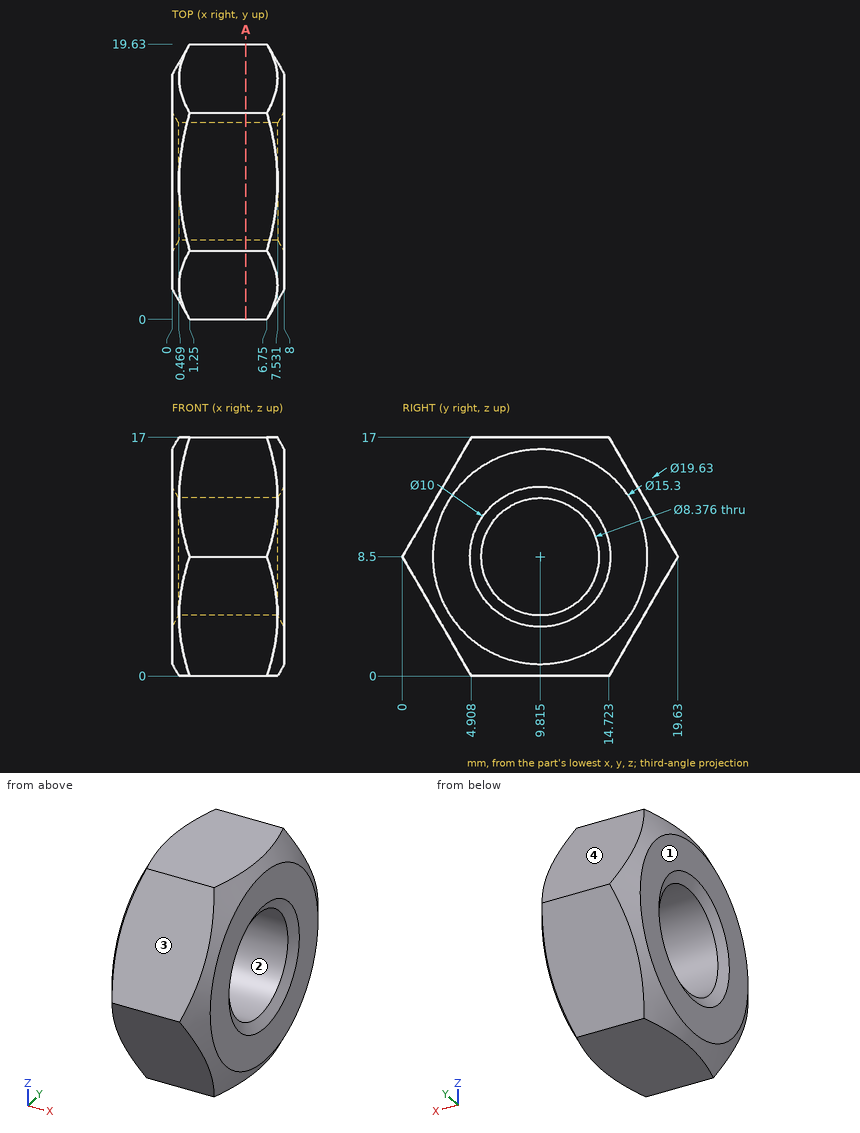
Geometry: see drawing. Coordinates: mm, zero at the bounding-box minimum. Coordinates: 2 decimals unless noted, no trailing zeros. Loops run counter-clockwise (first coordinate to the right, second up) from the corner with the lowest first, then second, coordinate; pieces in that order, holes last. Notation, with made-up numbers: (60.5, -4.5) - (88.5, -4.5) arc R28 cw to (88.5, 29.5) - close; hole circle Ø4 at (44, 46.5). An arc over 180 degrees is marked (long way). Answer in a Markdown table with one row per item.
(1) Pin query (flat end, axial travel): P1, Ø1, axis at x = 1, z = 8, coming from the +Y side. Return the tip coordinate at first contact, or that it passes through.
Model answer:
| item | result |
|---|---|
| P1 | stops at y = 19.6 |
(2) Cut plane A-A on x = 5.25. Output: boundary loops of the cut face in (y, z) (1 decimal), plus the area to 3 significant figures.
Model answer:
| item | result |
|---|---|
| outline | (0, 8.5) - (4.9, 0) - (14.7, 0) - (19.6, 8.5) - (14.7, 17) - (4.9, 17) - close; hole circle Ø8.4 at (9.8, 8.5) |
| area | 195 mm² |
(3) Mould query, pull axis Y, two halves, no side actions, for the marked faces 1, 2, 3 and 4. Classes: pulls with the +Y half, pulls with the -Y half, needs draft (parallel to the pull), parting line crosses it, or undercut.
Model answer:
| item | result |
|---|---|
| face 1 | needs draft |
| face 2 | undercut |
| face 3 | pulls with the -Y half |
| face 4 | pulls with the +Y half |
(4) Material intervals for L1, parallel to Y at x = 6.25, z = 5.5 (1 decimal); L2, parallel to Y at x = 4.75, z = 11 (1 decimal); L3, parallel to Z at x = 3.5, y = 7.5, sorted ascending. Write a range as from..to.
Model answer:
| item | result |
|---|---|
| L1 | y = 1.7..6.9, 12.7..17.9 |
| L2 | y = 1.4..6.5, 13.2..18.2 |
| L3 | z = 0..5.01, 11.99..17 |
